Input: part model. Units: mm. Frame: model coordinates. A direction names the side the tool comes from. Coordinates: 2 decimals unless noted, no trailing zeros. Loops run counter-clockwise (first coordinate to the right, second up) from the corner with the lowest first, then second, coordinate; pieces in that order, holes last.
Item 1: Pull-direction query (Y, two-part tool) for faces 1 (the flat face through (-92, -21, 42)), 2 (the flat face through (-88, 20, 42)), 3 (the flat face through (-6, 25, 24)), 4 (the flat face through (-4, -25, 24)); classes: released by +Y, released by -Y, zero draft, split by the parting line, or undercut.
Item 2: Ray query, line 1 along X through (y, z) = (-5.5, 29); line 2 along Y through (x, z) = (-81, 38). Return the intervals inside material, ascending.
Item 3: Reachability of faces 5 (the flat face through (-82, 0, 24)), 6 (the flat face through (-88, -20, 42)), 7 (the flat face through (-88, 21, 38)) from +Z, -Z, +X, -X, +Y, -Y: full face, straight path, thin tool, end or side. Return the list, or none.
Item 4: Section A-A on y = 11. Return loops of the section in (x, z), and give its area (3 significant figures).
Item 5: Section B-B on z = 10. Return loops of the section in (x, y), and give its area (3 significant figures).
Item 6: Contact query for flat-ended pins moving along their axis: P1, Ø1.5, axis at x = -88, y = -22, coming from the -Z side; P2, Ø22, axis at y = 0, z = 33.5, coming from the -X side. Output: stop coordinate, or through.
```python
from build123d import *

# Parameters (mm, degrees)
SKETCH1_W           = 164
SKETCH1_H           = 50
BOSS_EXTRUDE1_DEPTH = 48
SKETCH2_W           = 10
SKETCH2_H           = 5
BOSS_EXTRUDE2_DEPTH = 10
FILLET1_R           = 2


with BuildPart() as part:
    # Sketch1 → Boss-Extrude1 (new body)
    with BuildSketch(Plane.XY):
        Rectangle(SKETCH1_W, SKETCH1_H)
    extrude(amount=BOSS_EXTRUDE1_DEPTH)

    # Sketch2 → Boss-Extrude2 (add)
    with BuildSketch(Plane.ZY.offset(82)):
        with Locations((43, -22.5)):
            Rectangle(SKETCH2_W, SKETCH2_H)
        with Locations((43, 22.5)):
            Rectangle(SKETCH2_W, SKETCH2_H)
    extrude(amount=BOSS_EXTRUDE2_DEPTH)

    # Fillet1
    fillet1_edges = [part.edges().sort_by_distance(p)[0] for p in [
        (-82, 0, 48),
        (-82, 25, 19),
        (-82, 22.5, 38),
        (-87, 25, 38),
        (-5, -25, 48),
        (-82, 20, 43),
        (-87, 20, 48),
        (-92, 25, 43),
        (-92, 22.5, 48),
        (-82, -25, 19),
        (-82, -20, 43),
        (-87, -20, 48),
        (-82, -22.5, 38),
        (-87, -25, 38),
        (-92, -22.5, 48),
        (-92, -25, 43),
        (82, 0, 48),
        (0, -25, 0),
        (-82, 0, 0),
        (0, 25, 0),
        (82, 0, 0),
        (82, -25, 24),
        (82, 25, 24),
        (-5, 25, 48),
    ]]
    fillet(fillet1_edges, radius=FILLET1_R)


solid = part.part
```
Results found:
1. face 1: zero draft
1. face 2: undercut
1. face 3: released by +Y
1. face 4: released by -Y
2. line 1: x = -82 to 82
2. line 2: y = -24.96 to 24.96
3. face 5: -Z, -X
3. face 6: +Z, -Z, -X
3. face 7: -Z, -X, +Y, -Y
4. outline: (-82, 2) arc R2 ccw to (-80, 0) - (80, 0) arc R2 ccw to (82, 2) - (82, 46) arc R2 ccw to (80, 48) - (-80, 48) arc R2 ccw to (-82, 46) - close
4. area: 7,870 mm2
5. outline: (-82, -23) arc R2 ccw to (-80, -25) - (80, -25) arc R2 ccw to (82, -23) - (82, 23) arc R2 ccw to (80, 25) - (-80, 25) arc R2 ccw to (-82, 23) - close
5. area: 8,200 mm2
6. P1: stops at z = 38
6. P2: stops at x = -82
